from build123d import *
from build123d.topology import SkipClean

# Parameters (mm, degrees)
BOSS_EXTRUDE1_DEPTH     = 10
SKETCH1_3_R             = 50
BOSS_EXTRUDE2_DEPTH     = 37.5
BOSS_EXTRUDE3_DEPTH     = 15
BOSS_EXTRUDE4_DEPTH     = 37.5
BOSS_EXTRUDE5_DEPTH     = 35
CUT_EXTRUDE1_DEPTH      = 312.749097833
CUT_EXTRUDE1_DEPTH_BACK = 312.749097833
SKETCH12_R              = 32.5
SKETCH12_W              = 5
SKETCH12_H              = 95


with BuildPart() as part:
    # Sketch1 → Boss-Extrude1 (new, symmetric)
    with BuildSketch(Plane.XY):
        with BuildLine():
            Line((50, 145), (50, 80))
            ThreePointArc((50, 80), (26.568542495, 23.431457505), (-30, 0))
            Line((-30, 0), (-175, 0))
            Line((-175, 0), (-175, 50))
            Line((-175, 50), (-90, 50))
            ThreePointArc((-90, 50), (-61.715728753, 61.715728753), (-50, 90))
            Line((-50, 90), (-50, 145))
            Line((-50, 145), (50, 145))
        make_face()
    extrude(amount=BOSS_EXTRUDE1_DEPTH, both=True)

    # Sketch1_3 → Boss-Extrude2 (add, symmetric)
    with BuildSketch(Plane.XY):
        with Locations((0, 145)):
            Circle(SKETCH1_3_R)
    extrude(amount=BOSS_EXTRUDE2_DEPTH, both=True)

    # Sketch2 → Boss-Extrude3 (add, symmetric)
    with BuildSketch(Plane.XY):
        with BuildLine():
            ThreePointArc((-90, 50), (-61.715728753, 61.715728753), (-50, 90))
            Line((-50, 90), (-50, 145))
            Line((-50, 145), (-35, 145))
            Line((-35, 145), (-35, 90))
            ThreePointArc((-35, 90), (-51.109127035, 51.109127035), (-90, 35))
            Line((-90, 35), (-175, 35))
            Line((-175, 35), (-175, 50))
            Line((-175, 50), (-90, 50))
        make_face()
    extrude(amount=BOSS_EXTRUDE3_DEPTH, both=True)

    # Sketch2_3 → Boss-Extrude4 (add, symmetric)
    with SkipClean():  # the faces are left unmerged after this step: merging them gives an invalid solid
        with BuildSketch(Plane.XY):
            with BuildLine():
                Line((-30, 15), (-175, 15))
                Line((-175, 15), (-175, 0))
                Line((-175, 0), (-30, 0))
                ThreePointArc((-30, 0), (26.568542495, 23.431457505), (50, 80))
                Line((50, 80), (50, 145))
                Line((50, 145), (35, 145))
                Line((35, 145), (35, 80))
                ThreePointArc((35, 80), (15.961940777, 34.038059223), (-30, 15))
            make_face()
        extrude(amount=BOSS_EXTRUDE4_DEPTH, both=True)
    add(part.part.scale(1), mode=Mode.REPLACE)  # the faces are merged on a copy

    # Sketch4 → Revolve1 (revolve)
    with BuildSketch(Plane.XY, mode=Mode.PRIVATE) as revolve1_sk:
        Polygon((-175, 55), (-202.5, 55), (-202.5, 15), (-212.5, 15), (-212.5, 0), (-175, 0), align=None)
    revolve(revolve1_sk.sketch.rotate(Axis((-175, 0, 0), (0, 1, 0)), 270), axis=Axis((-175, 0, 0), (0, 1, 0)))

    # Sketch6 → Boss-Extrude5 (add, symmetric)
    with BuildSketch(Plane(origin=(0, 0, 0), x_dir=(0, 0, -1), z_dir=(1, 0, 0))):
        with BuildLine():
            Line((-25.325716562, 145), (25.325716562, 145))
            Line((25.325716562, 145), (19.923893962, 206.743114855))
            ThreePointArc((19.923893962, 206.743114855), (0, 225), (-19.923893962, 206.743114855))
            Line((-19.923893962, 206.743114855), (-25.325716562, 145))
        make_face()
    extrude(amount=BOSS_EXTRUDE5_DEPTH, both=True)

    # Sketch11 → CBORE for M12 SBHCS1 (revolve, cut)
    with BuildSketch(Plane(origin=(-35, 205, 0), x_dir=(0, 0, 1), z_dir=(0, 1, 0))):
        Polygon((0, 0), (0, 85), (6.75, 85), (6.75, 6.6), (11, 6.6), (11, 0.025), (11.025, 0), align=None)
    revolve(axis=Axis((-41.35, 205, 0), (1, 0, 0)), mode=Mode.SUBTRACT)

    # Sketch12 → Cut-Extrude1 (cut, two sides: drawn at the far end of the back side and taken through both)
    with BuildSketch(Plane.XY.offset(-CUT_EXTRUDE1_DEPTH_BACK)):
        with Locations((0, 145)):
            Circle(SKETCH12_R)
        with Locations((0, 177.5)):
            Rectangle(SKETCH12_W, SKETCH12_H)
    extrude(amount=CUT_EXTRUDE1_DEPTH + CUT_EXTRUDE1_DEPTH_BACK, mode=Mode.SUBTRACT)

    # Sketch13 → Cut-Revolve1 (revolve, cut)
    with BuildSketch(Plane.XY, mode=Mode.PRIVATE) as cut_revolve1_sk:
        Polygon((-175, 0), (-200, 0), (-200, 5), (-190, 5), (-190, 50), (-195, 50), (-195, 55), (-175, 55), align=None)
    revolve(cut_revolve1_sk.sketch.rotate(Axis((-175, 55, 0), (0, -1, 0)), 270), axis=Axis((-175, 55, 0), (0, -1, 0)), mode=Mode.SUBTRACT)


solid = part.part
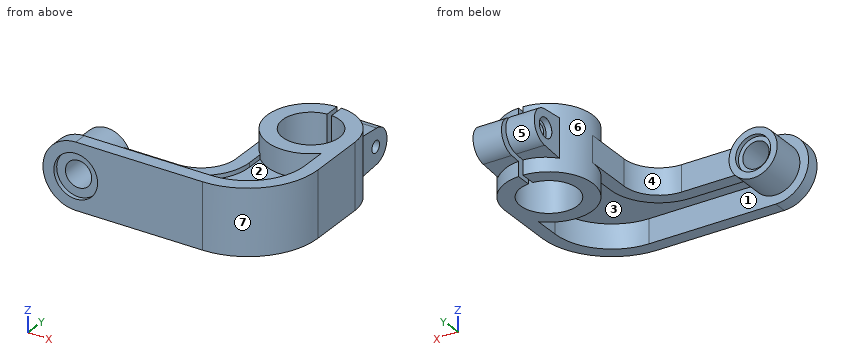
Could you check a few things on this model? Use its own coordinates, in mm. Face numbers are marked on the shaded views. A direction names the side the tool comes from. Coordinates: 2 decimals unless noted, no trailing zeros. Loops run counter-clockwise (first coordinate to the right, second up) from the corner with the lowest first, then second, coordinate; pieces in that order, holes last. Notation, with made-up numbers: (3, -37) -> (40, -37) arc R15 cw to (40, -21) -> close; hole circle Ø1 at (16, 26). An arc over 180 degrees is marked (long way). Answer in a Markdown table with one row per item.
(1) Imagine slicing it at B-B (y = 190). List the corners of the cut face in (x, z) for me.
Results found:
| item | result |
|---|---|
| outline | (-35, -21.39) -> (-21.79, -21.39) -> (-21.79, -37.5) -> (-2.5, -37.5) -> (-2.5, 37.5) -> (-21.79, 37.5) -> (-21.79, 21.39) -> (-35, 21.39) -> close; (2.5, -37.5) -> (21.79, -37.5) -> (21.79, -21.39) -> (35, -21.39) -> (35, 21.39) -> (21.79, 21.39) -> (21.79, 37.5) -> (2.5, 37.5) -> close |
(2) If I drill on probe 1 along X at (y, z) = (145, -14); probe 2 along Y at (x, z) = (6.5, 0); probe 3 along Y at (x, z) = (-59, -26), over which ranges is the centre line in solid material (lowest first)?
Results found:
| item | result |
|---|---|
| probe 1 | x = -50 to -32.5, 32.5 to 50 |
| probe 2 | y = 8.81 to 113.16, 176.84 to 198.25, 211.75 to 225 |
| probe 3 | y = 0 to 15 |
(3) Will these pins go through, and if not, where does the flat tip stop? pin 1 Ø25 at (x, z) = (-177, 8) entering from -Y; pin 2 Ø6.5 at (y, z) = (203.5, -1) entering from -X; pin 3 Ø2 at (x, z) = (11.5, 23) entering from +Y; pin 4 Ø2 at (y, z) = (30, 6) entering from +X.
Results found:
| item | result |
|---|---|
| pin 1 | stops at y = 5 |
| pin 2 | passes through |
| pin 3 | stops at y = 193.89 |
| pin 4 | stops at x = 33.24 |
(4) Imagine slicing it at C-C (z = 0). Give the number of separate pieces and of enclosed holes in the cut face, plus the area to 3 significant figures.
Results found:
| item | result |
|---|---|
| separate pieces | 4 |
| enclosed holes | 0 |
| area | 21,600 mm^2 |
(5) Imagine slicing it at D-D (y = 23.5). List the corners of the cut face in (x, z) for me, plus the area to 3 significant figures.
Results found:
| item | result |
|---|---|
| outline | (-149.38, -10) -> (2.14, -10) -> (2.14, -37.5) -> (26.64, -37.5) -> (26.64, 37.5) -> (2.14, 37.5) -> (2.14, 10) -> (-149.38, 10) arc R27.5 ccw (long way) to start; hole circle Ø30 at (-175, 0) |
| area | 6,510 mm^2 |
(6) Imagine slicing it at A-A (x = -126). List the corners of the cut face in (y, z) for me.
Results found:
| item | result |
|---|---|
| outline | (0, -37.5) -> (15, -37.5) -> (15, -10) -> (35, -10) -> (35, -15) -> (50, -15) -> (50, 15) -> (35, 15) -> (35, 10) -> (15, 10) -> (15, 37.5) -> (0, 37.5) -> close |
(7) Thinking about a two-plate mould opening in X: for the marked faces 5, 6 and 7, which applies, released by +X, released by -X, zero draft, split by the parting line, or undercut?
Results found:
| item | result |
|---|---|
| face 5 | zero draft |
| face 6 | undercut |
| face 7 | released by +X |
(8) For the marked faces 1, 2, 3 and 4, which set-ups out of +Z, -Z, +X, -X, +Y, -Y let a thin tool reach every point of the face, with its end or its side?
Results found:
| item | result |
|---|---|
| face 1 | none |
| face 2 | +Z |
| face 3 | -Z |
| face 4 | +Z, -Z, +Y |
